The listing builds one solid part. Answer for the finished solid, in the listing's coordinates (mm). Face numbers are marked on the shaded views. Give positions to 0.01 mm unless a question says otherwise; leave off trailing zeros. Order: outer loops, then holes, each group sorted by start corner. A loop starts at its lowest first (then second) coordinate and runs counter-clockwise, first axis right, second up. Notation, with made-up numbers: (76.5, 59) - (119.5, 59) arc R19 ccw to (119.5, 74) - close; hole circle Ø5 at (19.5, 56.5). An arc over 180 degrees is marked (long way). Answer in a Markdown table with one row per item.
from build123d import *

# Parameters (mm, degrees)
HEX_START         = -3.217333
HEX_2_DEPTH       = 3.217333
CHAMFER1_SIZE     = 0.381
FILLET1_R         = 0.1905
SKETCH3_R         = 2.291358881
HEX_CHAMFER_DEPTH = 2.54
HEX_CHAMFER_DRAFT = 45


with BuildPart() as part:
    # Sketch1 → Body (revolve)
    with BuildSketch(Plane(origin=(0, 0, 0), x_dir=(1, 0, 0), z_dir=(0, 1, 0))):
        Polygon((0, 0), (0, 3.9624), (4.826, 3.9624), (4.826, 2.413), (55.626, 2.413), (55.626, 0), align=None)
    revolve(axis=Axis((55.626, 0, 0), (-1, 0, 0)))

    # Sketch2 → Hex 2 (cut)
    with BuildSketch(Plane.ZY.offset(HEX_START)):
        Polygon((-2.291358881, 0), (-1.14567944, -1.984375), (1.14567944, -1.984375), (2.291358881, 0), (1.14567944, 1.984375), (-1.14567944, 1.984375), align=None)
    extrude(amount=HEX_2_DEPTH, mode=Mode.SUBTRACT)

    # Chamfer1
    chamfer1_edges = [part.edges().sort_by_distance(p)[0] for p in [
        (0, 0, 3.9624),
        (55.626, 0, 2.413),
    ]]
    chamfer(chamfer1_edges, length=CHAMFER1_SIZE)

    # Fillet1
    fillet1_edges = [part.edges().sort_by_distance(p)[0] for p in [
        (4.826, 0, 2.413),
    ]]
    fillet(fillet1_edges, radius=FILLET1_R)


with BuildPart() as hex_chamfer_tool:
    # Sketch3 → Hex Chamfer (with draft: the straight prism first)
    with BuildSketch(Plane(origin=(0, 0, 0), x_dir=(0, 0, -1), z_dir=(1, 0, 0))):
        Circle(SKETCH3_R)
    extrude(amount=HEX_CHAMFER_DEPTH)
    # Hex Chamfer: the draft: its side faces are tilted about the plane it starts from
    hex_chamfer_sides = [hex_chamfer_tool.faces().sort_by_distance(p)[0] for p in [
        (1.27, 0, 2.291358881),
    ]]
    draft(hex_chamfer_sides, Plane(origin=(0, 0, 0), x_dir=(0, 0, -1), z_dir=(1, 0, 0)), HEX_CHAMFER_DRAFT)


with BuildPart() as part_1:
    add(part.part)

    # Hex Chamfer: cut by hex_chamfer_tool
    add(hex_chamfer_tool.part, mode=Mode.SUBTRACT)


solid = part_1.part
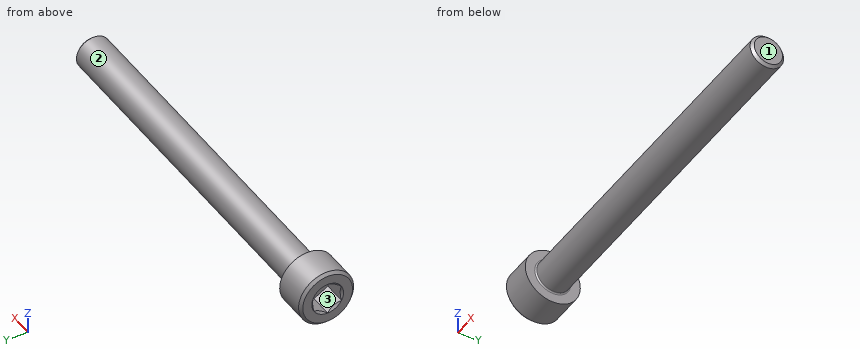
Item 1: Each of these flat-tipped pins is pushed along its axis until it touches: P1, Ø1, axis at x = 32, y = 1, coming from the +Z side; P2, Ø3, axis at y = -0.5, z = 0.5, coming from the -X side; P3, Ø3, axis at x = 19.5, y = -2.5, coming from the -Z side. Where does it stop, or does it pass through?
Answer block:
| item | result |
|---|---|
| P1 | z = 2.36 |
| P2 | x = 0.08 |
| P3 | z = -2.2 |
Item 2: Find section B-B on x = 8.5. Write down the section's boundary in (y, z), then the cut area to 3 significant figures.
Answer block:
| item | result |
|---|---|
| outline | circle Ø4.83 at (0, 0) |
| area | 18.3 mm² |
Item 3: Consider line 1 (X direction, y = -1.75, z = 2.25); line 2 (Y direction, x = 26, z = 0); line 3 (X direction, y = -0.75, z = 1). Determine where each line is inside the solid, lowest interval first.
Answer block:
| item | result |
|---|---|
| line 1 | 0 to 4.83 |
| line 2 | -2.41 to 2.41 |
| line 3 | 3.22 to 55.63 |
Item 4: Determine the mould class of the marked faces 1, 2 and 3 for opening direction Y: pulls with the +Y half, pulls with the -Y half, needs draft (parallel to the pull), parting line crosses it, or undercut.
Answer block:
| item | result |
|---|---|
| face 1 | needs draft |
| face 2 | parting line crosses it |
| face 3 | undercut |
